from build123d import *

# Parameters (mm, degrees)
SKETCH_1_R               = 30
EXTRUDE_1_DEPTH          = 26.3
SKETCH_2_R               = 22.5
CUT_EXTRUDE_1_DEPTH      = 27.3
SKETCH_3_R               = 8.5
SKETCH_3_R_2             = 2
EXTRUDE_2_DEPTH          = 8
CUT_EXTRUDE_2_DEPTH      = 6
EXTRUDE_3_DEPTH          = 3
PATTERN_CIRCULAR_1_COUNT = 7
FILLET_1_R               = 1


with BuildPart() as part:
    # Sketch 1 → Extrude 1 (new body)
    with BuildSketch(Plane.XY):
        Circle(SKETCH_1_R)
    extrude(amount=EXTRUDE_1_DEPTH)

    # Sketch 2 → Cut-Extrude 1 (cut, through all)
    with BuildSketch(Plane(origin=(0, 0, 0), x_dir=(-1, 0, 0), z_dir=(0, 0, -1))):
        Circle(SKETCH_2_R)
    extrude(amount=-CUT_EXTRUDE_1_DEPTH, mode=Mode.SUBTRACT)



with BuildPart() as body_2:
    # Sketch 3 → Extrude 2 (new body)
    with BuildSketch(Plane(origin=(0, 0, 10), x_dir=(-1, 0, 0), z_dir=(0, 0, -1))):
        Circle(SKETCH_3_R)
        Circle(SKETCH_3_R_2, mode=Mode.SUBTRACT)
    extrude(amount=-EXTRUDE_2_DEPTH)

    # Sketch 4 → Cut-Extrude 2 (cut)
    with BuildSketch(Plane(origin=(0, 0, 10), x_dir=(-1, 0, 0), z_dir=(0, 0, -1))):
        Polygon((7.216878365, 0), (3.608439182, 6.25), (-3.608439182, 6.25), (-7.216878365, 0), (-3.608439182, -6.25), (3.608439182, -6.25), align=None)
    extrude(amount=-CUT_EXTRUDE_2_DEPTH, mode=Mode.SUBTRACT)


with BuildPart() as part_1:
    add(part.part)

    add(body_2.part)  # Extrude 3 merges body 2
    # Sketch 5 → Extrude 3 (add, symmetric)
    with BuildSketch(Plane(origin=(0, 0, 0), x_dir=(1, 0, 0), z_dir=(0, 1, 0))):
        Polygon((-22.5, 0), (-15.275057212, 0), (-7.243077648, -10), (-8.396842229, -10), (-16.069885632, -2.529070305), (-24.164958171, -2.529070305), (-24.164958171, 0), align=None)
    extrude_3 = extrude(amount=EXTRUDE_3_DEPTH, both=True)

    # Pattern Circular 1: Extrude 3 ×7 about axis
    pattern_circular_1_axis = Axis((0, 0, 0), (0, 0, 1))
    for i in range(1, PATTERN_CIRCULAR_1_COUNT):
        add(extrude_3.rotate(pattern_circular_1_axis, i * 360 / PATTERN_CIRCULAR_1_COUNT))

    # Fillet 1
    fillet_1_edges = [part_1.edges().sort_by_distance(p)[0] for p in [
        (-30, 0, 0),
        (-30, 0, 26.3),
    ]]
    fillet(fillet_1_edges, radius=FILLET_1_R)


solid = part_1.part
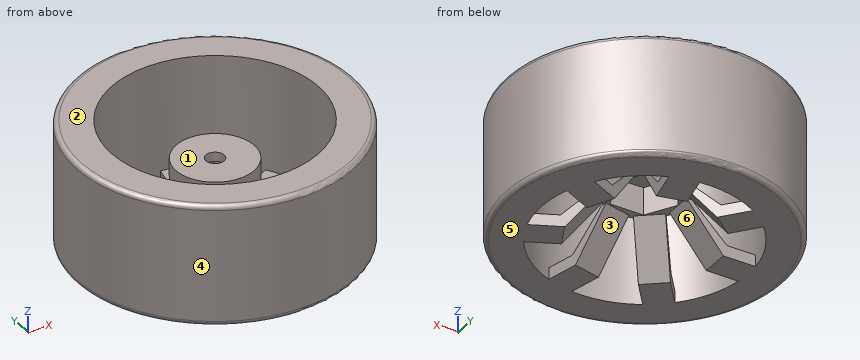
Check sheet for the modelled part. Datum: model origin and axes. Units: mm. Face numbers are marked on the shaded views. A direction names the side the tool comes from. Give positions to 0.01 mm unless a question says otherwise; leave off trailing zeros. Write each loop counter-clockwise with the first axis right and the second up, starting at its lowest first coordinate (ties: lowest second). Pieces come first, ordered by that corner, then holes. Notation, with made-up numbers: M 13.5,17 L 24.5,17 A7 cw 24.5,23 Z; hole C 8.25,37 d9. An arc over 180 degrees is marked long. Use one line per item in the form item = value.
(1) Depth check by flat-ended pin: P1, Ø2.5, axis at x = 17, y = 9, coming from the +Z side; P2, Ø1.3, axis at x = 7.5, y = 3.5, coming from the -Z side; P3, Ø0.5, axis at x = 0, y = 8.5, coming from the +Z side. Enter the tip coordinate at first touch or a pass-through.
Answer block:
P1 = 2.53
P2 = 7.9
P3 = 18
(2) Material ranges on line 1 along Y through (x, z) = (0, 16.85); line 2 along Y through (x, z) = (0, 14.5); line 3 along X through (y, z) = (2, 20.75), recorded low to high.
Answer block:
line_1 = -30 to -22.5, -8.5 to -2, 2 to 8.5, 22.5 to 30
line_2 = -30 to -22.5, -8.5 to -6.25, 6.25 to 8.5, 22.5 to 30
line_3 = -29.93 to -22.41, 22.41 to 29.93
(3) Section check B-B on z = 4. State how many separate pieces and enclosed holes the cut face has, plus the area to 3 significant figures.
Answer block:
separate_pieces = 8
enclosed_holes = 1
area = 1,340 mm2
(4) Tool access check on the marked faces 1, 2 and 3. Record the directions out of +Z, -Z, +X, -X, +Y, -Y that give a thin tool (end or side, any length) a straight path to the whole face; none if there is none.
Answer block:
face_1 = +Z
face_2 = +Z, +X, -X, +Y, -Y
face_3 = -Z
(5) Section check A-A on z = 13.25. Record the boundary of the cut face in (x, y), plus the area to 3 significant figures.
Answer block:
outline = C 0,0 d60; C 0,0 d17; hole C 0,0 d45; hole M -7.22,0 L -3.61,-6.25 L 3.61,-6.25 L 7.22,0 L 3.61,6.25 L -3.61,6.25 Z
area = 1,330 mm2
(6) Draft check along X on the marked faces 4, 5 and 6. Enter one of: pulls with the +X half, pulls with the -X half, needs draft (parallel to the pull), parting line crosses it, or undercut.
Answer block:
face_4 = parting line crosses it
face_5 = needs draft
face_6 = undercut
